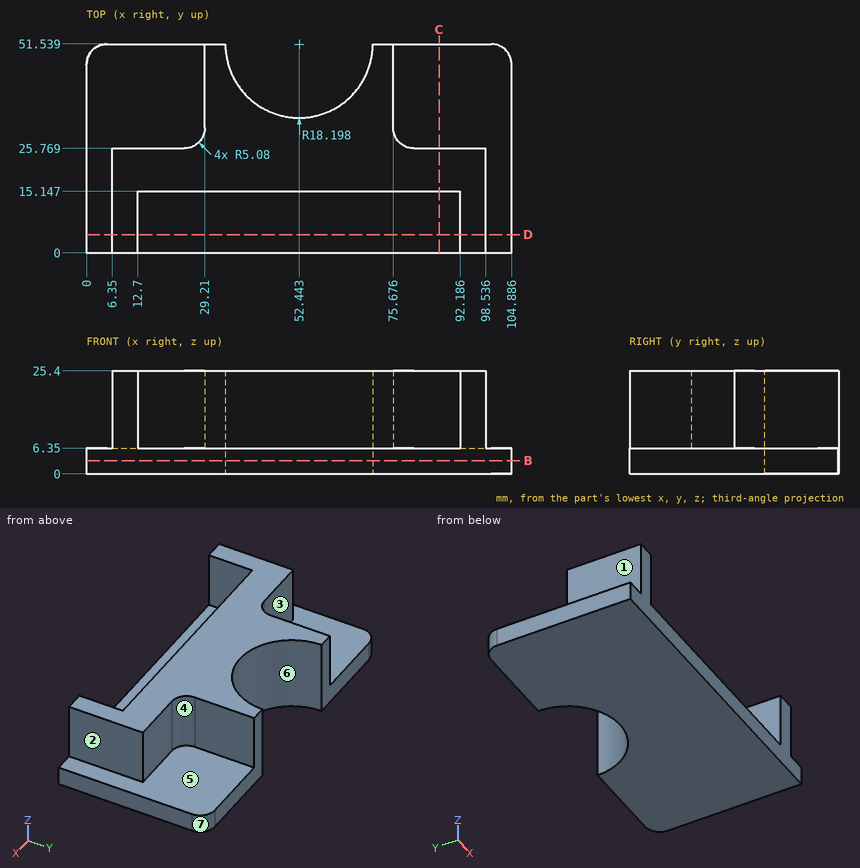
Could you check a few things on this drawing? It's one solid part, dimensions in mm from its lowest x, y, z. A direction names the side the tool comes from. Round coordinates to 2 decimals unless told otherwise and drop trailing zeros. Write each loop counter-clockwise with the first axis right and the second up, starting at its lowest first coordinate (ties: lowest second). Pieces come first, ordered by that corner, then holes.
Q1. If we section it at C-C on x = 87: Write out the boundary of the cut face in (y, z).
Q2. If we mould it in two halves opening along X, with no side actions, what happens to the marked faces 5, 6 and 7? For each: +X half, -X half, draft (parallel to the pull), parting line (faces both ways), or undercut.
Q3. Will these pins go through, and if not, where does the flat tip stop? P1, Ø7.5, axis at y = 11.5, z = 19.5, coming from the +X side; P2, Ø15, axis at y = 44, z = 19.5, coming from the +X side; P3, Ø1, axis at x = 25.5, z = 18, coming from the -Y side; P4, Ø23.5, axis at x = 94, y = 28.5, coming from the +Z side.
Q4. If we section it at B-B on z = 3.25: Write out the boundary of the cut face in (x, y) (1 decimal).
Q5. If we section it at D-D on y = 4.5: Write out the boundary of the cut face in (x, z), plus the area to 3 significant figures.
Q6. Which directions (+Z, -Z, +X, -X, +Y, -Y) give clear straight access to the entire face, cutting with the end or side of a thin tool? Please do the marked faces 1, 2, 3 and 4.
Q7. Please list where these lines run through material, in increasing order: probe 1 along X at (y, z) = (9.5, 17.5); probe 2 along Y at (x, z) = (21, 14.5); probe 3 along X at (y, z) = (49, 21.75).
Answer below:
1. outline: (0, 0) - (51.54, 0) - (51.54, 6.35) - (25.77, 6.35) - (25.77, 25.4) - (15.15, 25.4) - (15.15, 6.35) - (0, 6.35) - close
2. face 5: draft
2. face 6: undercut
2. face 7: +X half
3. P1: stops at x = 98.54
3. P2: stops at x = 75.68
3. P3: stops at y = 15.15
3. P4: stops at z = 25.4
4. outline: (0, 0) - (104.9, 0) - (104.9, 46.5) arc R5.1 ccw to (99.8, 51.5) - (70.6, 51.5) arc R18.2 cw to (34.2, 51.5) - (5.1, 51.5) arc R5.1 ccw to (0, 46.5) - close
5. outline: (0, 0) - (104.89, 0) - (104.89, 6.35) - (98.54, 6.35) - (98.54, 25.4) - (92.19, 25.4) - (92.19, 6.35) - (12.7, 6.35) - (12.7, 25.4) - (6.35, 25.4) - (6.35, 6.35) - (0, 6.35) - close
5. area: 908 mm2
6. face 1: +Z, -X, +Y, -Y
6. face 2: +Z, +X, +Y, -Y
6. face 3: +Z, -X, +Y
6. face 4: +Z, +X, +Y
7. probe 1: x = 6.35 to 12.7, 92.19 to 98.54
7. probe 2: y = 15.15 to 25.77
7. probe 3: x = 29.21 to 34.42, 70.46 to 75.68
